Work out the finished part from the listing and answer in its coordinate system (mm). Face numbers are marked on the shaded views. A direction names the side the tool comes from. Round coordinates to 2 decimals unless told otherwise and drop trailing zeros. Order: outer loops, then holes, each group sorted by start corner. A loop starts at its lowest first (then second) coordinate and runs counter-clockwise, first axis right, second up. Notation, with made-up numbers: (56.5, 54) -> (86.5, 54) arc R15 cw to (86.5, 67) -> close; hole circle Ø6 at (3.5, -2). An arc over 180 degrees is marked (long way). Use a Markdown table: item, result. Add a question column.
Item 1: A cutting plane is placed at A-A, the plane x = 15. Determine the outline of the cut face in (y, z), plus the area to 3 significant figures.
Item 2: A cutting plane is placed at B-B, the plane z = -15. Determine the outline of the cut face in (x, y), plus the area to 3 significant figures.
Item 3: A cutting plane is placed at D-D, the plane z = -7.5. Determine the outline of the cut face in (x, y), plus the area to 3 significant figures.
Item 4: A cutting plane is placed at C-C, the plane y = 15. Determine the outline of the cut face in (x, z), plus the area to 3 significant figures.
Item 5: Flat-ended cylindrical pins translate along their axes: P1, Ø7, axis at x = 15, z = -15, coming from the +Y side; P2, Ø14.5, axis at x = 12, z = -16, coming from the +Y side; P3, Ø4.5, axis at y = 40.054, z = -7.5, coming from the -X side; P4, Ø3, axis at y = 24, z = -18.5, coming from the +X side. Find the tip coordinate at first contact, or state that the pin passes through.
Item 6: Find the intervals of material crossed by L1, parallel to Y at x = -5.5, z = -7.5; L2, parallel to X at y = 6.9, z = -15; L3, parallel to Y at x = -7, z = -8.75, in increasing order. Write a range as [from, to].
Item 7: A tool of negligible diameter and unlimited length cuts with its end or side. For the marked faces 5, 6 and 7, from which of +Z, -Z, +X, -X, +Y, -Y can it reach the whole face along a straight path? Write none if from no direction.
Item 8: For a pull along X with two mould halves and no side action, classify the marked faces 1, 2, 3 and 4 as +X half, -X half, draft (parallel to the pull), parting line (faces both ways), or undercut.
from build123d import *

# Parameters (mm, degrees)
SKETCH3_W           = 30
SKETCH3_H           = 30
BOSS_EXTRUDE2_DEPTH = 17.544106429
SKETCH8_R           = 14
CUT_EXTRUDE1_DEPTH  = 9.554
SKETCH9_R           = 9
CUT_EXTRUDE2_DEPTH  = 2
SKETCH10_R          = 3
CUT_EXTRUDE3_DEPTH  = 44.971523922
SKETCH13_W          = 30
SKETCH13_H          = 47.544106429
BOSS_EXTRUDE3_DEPTH = 13.972846029
SKETCH14_R          = 1.7
CUT_EXTRUDE4_DEPTH  = 64.721598035


with BuildPart() as part:
    # Sketch3 → Boss-Extrude2 (new body)
    with BuildSketch(Plane(origin=(0, 0, 0), x_dir=(1, 0, 0), z_dir=(0, 1, 0))):
        with Locations((15, 15)):
            Rectangle(SKETCH3_W, SKETCH3_H)
    extrude(amount=BOSS_EXTRUDE2_DEPTH)

    # Sketch8 → Cut-Extrude1 (cut)
    with BuildSketch(Plane(origin=(0, 17.544106429, 0), x_dir=(1, 0, 0), z_dir=(0, 1, 0))):
        with Locations(Location((15, 15, 0), (0, 0, 270))):
            Circle(SKETCH8_R)
    extrude(amount=-CUT_EXTRUDE1_DEPTH, mode=Mode.SUBTRACT)

    # Sketch9 → Cut-Extrude2 (cut)
    with BuildSketch(Plane(origin=(0, 7.990106429, 0), x_dir=(1, 0, 0), z_dir=(0, 1, 0))):
        with Locations(Location((15, 15, 0), (0, 0, 270))):
            Circle(SKETCH9_R)
    extrude(amount=-CUT_EXTRUDE2_DEPTH, mode=Mode.SUBTRACT)

    # Sketch10 → Cut-Extrude3 (cut, through all)
    with BuildSketch(Plane(origin=(0, 5.990106429, 0), x_dir=(1, 0, 0), z_dir=(0, 1, 0))):
        with Locations(Location((15, 15, 0), (0, 0, 270))):
            Circle(SKETCH10_R)
    extrude(amount=-CUT_EXTRUDE3_DEPTH, mode=Mode.SUBTRACT)

    # Sketch13 → Boss-Extrude3 (add)
    with BuildSketch(Plane.ZY):
        with Locations((-15, 23.772053215)):
            Rectangle(SKETCH13_W, SKETCH13_H)
    extrude(amount=BOSS_EXTRUDE3_DEPTH)

    # Sketch14 → Cut-Extrude4 (cut, through all)
    with BuildSketch(Plane(origin=(0, 0, 0), x_dir=(0, 0, -1), z_dir=(1, 0, 0))):
        with Locations((7.5, 25.054)):
            Circle(SKETCH14_R)
        with Locations((7.5, 40.054)):
            Circle(SKETCH14_R)
        with Locations((22.5, 25.054)):
            Circle(SKETCH14_R)
        with Locations((22.5, 40.054)):
            Circle(SKETCH14_R)
    extrude(amount=-CUT_EXTRUDE4_DEPTH, mode=Mode.SUBTRACT)


solid = part.part
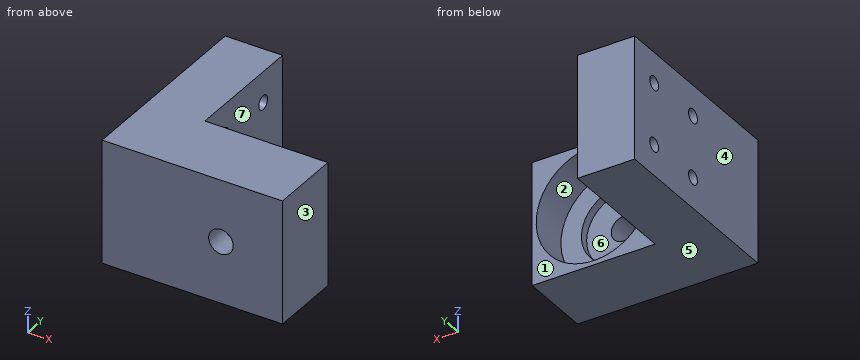
Reported:
| question | item | result |
|---|---|---|
| 1 | outline | (0, -30) -> (17.54, -30) -> (17.54, -29) -> (7.99, -29) -> (7.99, -24) -> (5.99, -24) -> (5.99, -18) -> (0, -18) -> close; (0, -12) -> (5.99, -12) -> (5.99, -6) -> (7.99, -6) -> (7.99, -1) -> (17.54, -1) -> (17.54, 0) -> (0, 0) -> close |
| 1 | area | 187 mm² |
| 2 | outline | (-13.97, 0) -> (12, 0) -> (12, 5.99) -> (6, 5.99) -> (6, 7.99) -> (1, 7.99) -> (1, 17.54) -> (0, 17.54) -> (0, 47.54) -> (-13.97, 47.54) -> close; (18, 0) -> (30, 0) -> (30, 17.54) -> (29, 17.54) -> (29, 7.99) -> (24, 7.99) -> (24, 5.99) -> (18, 5.99) -> close |
| 2 | area | 851 mm² |
| 3 | outline | (-13.97, 0) -> (30, 0) -> (30, 17.54) -> (26.82, 17.54) -> (26.82, 7.99) -> (19.97, 7.99) -> (19.97, 5.99) -> (10.03, 5.99) -> (10.03, 7.99) -> (3.18, 7.99) -> (3.18, 17.54) -> (0, 17.54) -> (0, 23.35) -> (-13.97, 23.35) -> close; (-13.97, 26.75) -> (0, 26.75) -> (0, 38.35) -> (-13.97, 38.35) -> close; (-13.97, 41.75) -> (0, 41.75) -> (0, 47.54) -> (-13.97, 47.54) -> close |
| 3 | area | 850 mm² |
| 4 | outline | (-13.97, -30) -> (30, -30) -> (30, 0) -> (-13.97, 0) -> close; hole circle Ø28 at (15, -15) |
| 4 | area | 703 mm² |
| 5 | P1 | y = 5.99 |
| 5 | P2 | y = 7.99 |
| 5 | P3 | x = -13.97 |
| 5 | P4 | x = 0 |
| 6 | L1 | [0, 23.35], [26.75, 38.35], [41.75, 47.54] |
| 6 | L2 | [-13.97, 6], [24, 30] |
| 6 | L3 | [0, 23.9], [26.21, 38.9], [41.21, 47.54] |
| 7 | face 5 | -Z, +X, -X, +Y, -Y |
| 7 | face 6 | +Y |
| 7 | face 7 | +Z, -Z, +X, +Y |
| 8 | face 1 | draft |
| 8 | face 2 | undercut |
| 8 | face 3 | +X half |
| 8 | face 4 | -X half |
